Geometry: final body of the model. Coordinates: model frame, mm. A direction names the side the tool comes from. Round coordinates to 2 decimals unless told otherwise and drop trailing zeros. Loops run counter-clockwise (first coordinate to the right, second up) from the corner with the lowest first, then second, coordinate; pieces in that order, holes last. Notation, with made-up numbers: (31.25, 67) - (86.25, 67) arc R28 cw to (86.25, 86) - close; hole circle Ø7 at (86, -20.75). An arc over 180 degrees is marked (long way). Return JSON: item names as keys, results as strings. Group by question number.
1. Section B-B on x = 20.25. Return loops of the section in (y, z), and give its area (3 significant figures).
2. Section C-C on z = 14.5. Return loops of the section in (x, y).
3. First-contact query: pin 1 Ø1.5 at (y, z) = (-7.5, 10.5) entering from +X. Flat tip, straight axial feed; report the tip coordinate or a pass-through.
4. Section A-A on y = -1. Return loops of the section in (x, z), and give its area (3 significant figures).
5. Section D-D on x = 17. Return loops of the section in (y, z).
6. Set-up query: faces 4 (the face through (15.614, -0.584, 3.425)), 5 (the face through (12.3, -4.5, 12.3)). Return all of +Z, -Z, +X, -X, +Y, -Y with unobstructed straight access to the full face (end or side cutting, diameter ignored); none if empty.
7. Draft query along X for faces 1 (the face through (-2.255, 0, 13)), 2 (the face through (4, 3, 12)), 3 (the face through (15.614, -6.11, 3.425)). Return one class per face: +X half, -X half, draft (parallel to the pull), parting line (faces both ways), or undercut.
8. Material intervals for probe 1 along Z at (x, y) = (8, -6.1); probe 2 along X at (y, z) = (0.5, 4.5); probe 3 along X at (y, z) = (-2, 4), sorted ascending.
from build123d import *

# Parameters (mm, degrees)
F0_W     = 25
F0_H     = 3
F1_DEPTH = 25
F3_DEPTH = 25
F4_R     = 1.5
F5_DEPTH = 25
F8_DEPTH = 25


with BuildPart() as f1:
    # F0 (on Top) → F1 (new body)
    with BuildSketch(Plane.XY):
        with Locations((12.5, 1.5)):
            Rectangle(F0_W, F0_H)
        with BuildLine():
            Line((25, 0), (0, 0))
            ThreePointArc((0, 0), (12.5, -4.5), (25, 0))
        make_face()
    extrude(amount=F1_DEPTH)


with BuildPart() as f3:
    # F2 (on face) → F3 (new body)
    with BuildSketch(Plane.XY.offset(25)):
        Polygon((-2.254958, -0.308215), (-0.254958, -0.308215), (-0.254958, 0), (0, 0), (0, 3), (-2.254958, 3), align=None)
        with BuildLine():
            ThreePointArc((25.254958, -0.308215), (12.5, -4.9), (-0.254958, -0.308215))
            Line((-0.254958, -0.308215), (-2.254958, -0.308215))
            Line((-2.254958, -0.308215), (-2.254958, -3.321898))
            ThreePointArc((-2.254958, -3.321898), (12.5, -8.5), (27.254958, -3.321898))
            Line((27.254958, -3.321898), (27.254958, -0.308215))
            Line((27.254958, -0.308215), (25.254958, -0.308215))
        make_face()
        Polygon((25.254958, 0), (25.254958, -0.308215), (27.254958, -0.308215), (27.254958, 3), (25, 3), (25, 0), align=None)
    extrude(amount=-F3_DEPTH)


with BuildPart() as f5_tool:
    # F4 (on face) → F5 (new body)
    with BuildSketch(Plane(origin=(0, 3, 0), x_dir=(-1, 0, 0), z_dir=(0, 1, 0))):
        with Locations((-17, 4)):
            Circle(F4_R)
        with Locations((-8, 4)):
            Circle(F4_R)
    extrude(amount=-F5_DEPTH)


with BuildPart() as f1_1:
    add(f1.part)

    # F5: cut by f5_tool
    add(f5_tool.part, mode=Mode.SUBTRACT)


with BuildPart() as f3_1:
    add(f3.part)

    # F5: cut by f5_tool
    add(f5_tool.part, mode=Mode.SUBTRACT)

    # F6: union F1
    add(f1_1.part)

    # F7 (on face) → F8 (cut)
    with BuildSketch(Plane(origin=(0, 0, 0), x_dir=(1, 0, 0), z_dir=(0, 0, -1))):
        with BuildLine():
            Line((12.5, 0), (12.5, -3))
            Line((12.5, -3), (15.5, -3))
            ThreePointArc((15.5, -3), (14.62132, -0.87868), (12.5, 0))
        make_face()
        with BuildLine():
            Line((9.5, -3), (12.5, -3))
            Line((12.5, -3), (12.5, 0))
            ThreePointArc((12.5, 0), (10.37868, -0.87868), (9.5, -3))
        make_face()
    extrude(amount=-F8_DEPTH, mode=Mode.SUBTRACT)


solid = f3_1.part
Taken from the geometry:
{
 "1": {"outline": "(-7.19, 0) - (-3.34, 0) - (-3.34, 25) - (-7.19, 25) - close; (-2.9, 0) - (3, 0) - (3, 25) - (-2.9, 25) - close", "area": "244 mm2"},
 "2": {"outline": "(-2.25, -3.32) arc R23.61 ccw to (27.25, -3.32) - (27.25, 3) - (15.5, 3) arc R3 cw to (12.5, 0) arc R3 cw to (9.5, 3) - (-2.25, 3) - close; hole (-0.25, -0.31) arc R20.01 ccw to (25.25, -0.31) - (25.25, 0) - (25, 0) arc R19.61 cw to (0, 0) - (-0.25, 0) - close"},
 "3": {"pin 1": "x = 21.42"},
 "4": {"outline": "(-2.25, 0) - (0.63, 0) - (0.63, 25) - (-2.25, 25) - close; (1.32, 0) - (23.68, 0) - (23.68, 25) - (1.32, 25) - close; (24.37, 0) - (27.25, 0) - (27.25, 25) - (24.37, 25) - close; hole circle Ø3 at (8, 4); hole circle Ø3 at (17, 4)", "area": "689 mm2"},
 "5": {"outline": "(-8.07, 0) - (-4.39, 0) - (-4.39, 2.5) - (-8.07, 2.5) - close; (-8.07, 5.5) - (-4.39, 5.5) - (-4.39, 25) - (-8.07, 25) - close; (-3.98, 0) - (3, 0) - (3, 2.5) - (-3.98, 2.5) - close; (-3.98, 5.5) - (3, 5.5) - (3, 25) - (-3.98, 25) - close"},
 "6": {"face 4": "+Y, -Y", "face 5": "+Z, -Z"},
 "7": {"face 1": "-X half", "face 2": "draft", "face 3": "undercut"},
 "8": {"probe 1": "0 to 2.5, 5.5 to 25", "probe 2": "-2.25 to 6.59, 9.41 to 10.84, 14.16 to 15.59, 18.41 to 27.25", "probe 3": "-2.25 to 2.12, 2.92 to 6.5, 9.5 to 15.5, 18.5 to 22.08, 22.88 to 27.25"}
}
